Read the model definition and answer for the solid it produces. Units are mm, in the model's axes. Round coordinates to 2 decimals unless told otherwise and drop trailing zeros. One line per item, written item: value. Start each with the question number.
1. Section A-A (z = -21) is taken. State how many separate pieces and enclosed holes the cut face has, then the cut area to 3 significant figures.
2. Flat-ended cylindrical pins translate along their axes: pin 1 Ø3 at (y, z) = (-292.1, -12.7) entering from -X; pin 2 Ø3 at (y, z) = (-285, -13.5) entering from -X. Find the tip coordinate at first contact, or state that the pin passes through.
3. Consider line 1 (Y direction, x = 6.5, z = 10.5); line 2 (Z direction, x = 4, y = -88.9); line 3 (Y direction, x = 6.35, z = -20). Determine where each line is inside the solid, lowest interval first.
from build123d import *

# Parameters (mm, degrees)
SKETCH1_W                                   = 12.7
SKETCH1_H                                   = 406.4
BOSS_EXTRUDE1_DEPTH                         = 25.4
F_10_32_THREADED_HOLES_D                    = 3.51028
CBORE_FOR_10_HEX_MACHINE_SCREW1_D           = 6.35
CBORE_FOR_10_HEX_MACHINE_SCREW1_CBORE_D     = 9.525
CBORE_FOR_10_HEX_MACHINE_SCREW1_CBORE_DEPTH = 12.7


with BuildPart() as part:
    # Sketch1 → Boss-Extrude1 (new, symmetric)
    with BuildSketch(Plane.XY):
        with Locations((6.35, -203.2)):
            Rectangle(SKETCH1_W, SKETCH1_H)
    extrude(amount=BOSS_EXTRUDE1_DEPTH, both=True)

    # #10-32 Threaded Holes (through all)
    with Locations(Plane(origin=(12.7, 0, 0), x_dir=(0, 0, -1), z_dir=(1, 0, 0))):
        with Locations((-12.7, -12.7), (12.7, -12.7), (-12.7, -38.1), (12.7, -38.1), (-12.7, -63.5), (12.7, -63.5), (-12.7, -88.9), (12.7, -88.9), (-12.7, -114.3), (12.7, -114.3), (-12.7, -139.7), (12.7, -139.7), (-12.7, -165.1), (12.7, -165.1), (-12.7, -190.5), (12.7, -190.5), (-12.7, -215.9), (12.7, -215.9), (-12.7, -241.3), (12.7, -241.3), (-12.7, -266.7), (12.7, -266.7), (-12.7, -292.1), (12.7, -292.1), (-12.7, -317.5), (12.7, -317.5), (-12.7, -342.9), (12.7, -342.9)):
            Hole(F_10_32_THREADED_HOLES_D / 2)

    # CBORE for #10 Hex Machine Screw1 (through all)
    with Locations(Plane(origin=(0, 0, -25.4), x_dir=(-1, 0, 0), z_dir=(0, 0, -1))):
        with Locations((-6.35, -396.24), (-6.35, -386.08), (-6.35, -375.92), (-6.35, -365.76)):
            CounterBoreHole(CBORE_FOR_10_HEX_MACHINE_SCREW1_D / 2, CBORE_FOR_10_HEX_MACHINE_SCREW1_CBORE_D / 2, CBORE_FOR_10_HEX_MACHINE_SCREW1_CBORE_DEPTH)


solid = part.part
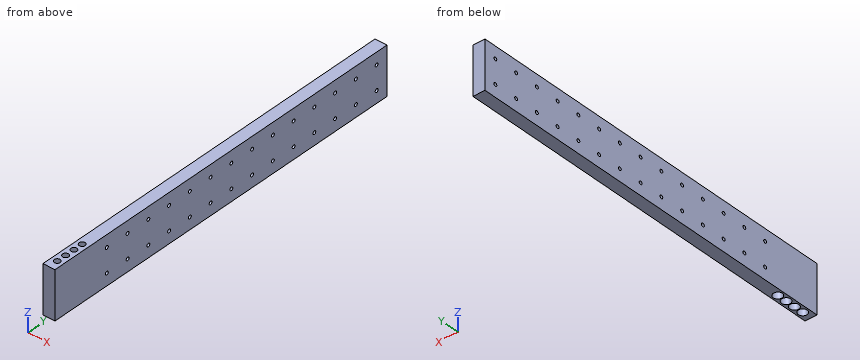
Answer:
1. separate pieces: 1
1. enclosed holes: 4
1. area: 4,880 mm^2
2. pin 1: through
2. pin 2: x = 0
3. line 1: -406.4 to -399.41, -393.07 to -389.25, -382.91 to -379.09, -372.75 to -368.93, -362.59 to 0
3. line 2: -25.4 to -14.46, -10.94 to 10.94, 14.46 to 25.4
3. line 3: -406.4 to -401, -391.48 to -390.84, -381.32 to -380.68, -371.16 to -370.52, -361 to 0
